Autodesk Inventor part; units mm, degrees
ref_plane "YZ Plane" through (0, 0, 0) normal (1, 0, 0) x (0, 1, 0)
ref_plane "XZ Plane" through (0, 0, 0) normal (0, 1, 0) x (-1, 0, 0)
ref_plane "XY Plane" through (0, 0, 0) normal (0, 0, 1) x (1, 0, 0)
sketch "Sketch2" plane through (0, 0, 0) normal (0, 1, 0) x (-1, 0, 0)
  line L0 (-49, 47) -> (-20, 47) construction
  line L1 (49, 47) -> (49, -47) construction
  line L2 (49, -47) -> (-49, -47)
  line L3 (-49, -47) -> (-49, 47) construction
  line L4 (-49, 47) -> (49, -47) construction
  line L5 (49, 47) -> (-49, -47) construction
  line L6 (49, -23) -> (45, -23)
  line L7 (45, -23) -> (45, 27)
  line L8 (45, 27) -> (49, 27)
  line L9 (49, 27) -> (49, -23)
  line L10 (-49, -23) -> (-45, -23)
  line L11 (-45, -23) -> (-45, 27)
  line L12 (-45, 27) -> (-49, 27)
  line L13 (-49, 27) -> (-49, -23)
  line L14 (25, -47) -> (-25, -47)
  line L15 (-25, -47) -> (-25, -43)
  line L16 (-25, -43) -> (25, -43)
  line L17 (25, -43) -> (25, -47)
  line L18 (0, -47) -> (0, 47)
  line L19 (49, 0) -> (-49, 0)
  line L20 (49, 2) -> (-45, 2) construction
  line L21 (20, 47) -> (0, 47) construction
  line L22 (-20, 47) -> (-20, 51) construction
  line L23 (-20, 51) -> (20, 51) construction
  line L24 (20, 51) -> (20, 47) construction
  line L25 (-20, 47) -> (20, 47)
  line L26 (0, 47) -> (-20, 47) construction
  line L27 (20, 47) -> (49, 47) construction
  line L28 (49, 43) -> (20, 43)
  line L29 (20, 43) -> (20, 47)
  line L30 (-49, 43) -> (-20, 43)
  line L31 (-20, 43) -> (-20, 47)
  line L32 (49, 43) -> (49, 27)
  line L33 (-49, 43) -> (-49, 27)
  line L34 (-49, -23) -> (-49, -47)
  line L35 (49, -23) -> (49, -47)
  point P0 (0, 0)
  point P1 (49, 27)
  point P2 (-49, 27)
  point P3 (0, 0)
  point P4 (0, 0)
  dimension "d7" = 98
  dimension "d8" = 94
  dimension "d5" = 4
  dimension "d6" = 50
  dimension "d3" = 4
  dimension "d4" = 50
  dimension "d1" = 50
  dimension "d2" = 4
  dimension "d0" = 2
  dimension "d27" = 4
  dimension "d28" = 40
  dimension "d31" = 4
extrude "Extrusion1" add sketch "Sketch2" along normal blind 4 contours L2 L17 L16 L18 L19 L7 L6 L35 | L2 L34 L10 L11 L19 L18 L16 L15 | L19 L18 L25 L29 L28 L32 L8 L7 | L19 L11 L12 L33 L30 L31 L25 L18
sketch "Sketch3" plane through (0, 4, 0) normal (0, 1, 0) x (1, 0, 0)
  circle A0 centre (0, 62.5) radius 11
  spline S0 degree 2 poles (-49, 47) (0, 109) (49, 47) knots 0 0 0 1 1 1
  circle A1 centre (66, -2) radius 7.5
  spline S1 degree 2 poles (49, 47) (117.0544, -3.4606) (49, -43) knots 0 0 0 1 1 1
  line L0 (0, 43) -> (0, -53.479) construction
  circle A2 centre (-66, -2) radius 7.5
  spline S2 degree 2 poles (-49, 47) (-117.0544, -3.4606) (-49, -43) knots 0 0 0 1 1 1
  line L1 (-66, 27) -> (-63.1716, 24.1716)
  line L2 (-63.1716, 24.1716) -> (-67.4142, 19.9289)
  line L3 (-67.4142, 19.9289) -> (-70.2426, 22.7574)
  line L4 (-70.2426, 22.7574) -> (-66, 27)
  line L5 (-20, -47) -> (-20, -51)
  line L6 (-20, -51) -> (20, -51)
  line L7 (20, -51) -> (20, -47)
  line L8 (49, 47) -> (25, 47) construction
  line L9 (25, 47) -> (25, 43)
  line L10 (25, 43) -> (-25, 43)
  line L11 (-25, 43) -> (-25, 47)
  line L12 (-25, 47) -> (-49, 47) construction
  line L13 (-49, 47) -> (-49, 23) construction
  line L14 (-49, 23) -> (-45, 23)
  line L15 (-45, 23) -> (-45, -27)
  line L16 (-45, -27) -> (-49, -27)
  line L17 (-49, -27) -> (-49, -43) construction
  line L18 (-49, -43) -> (-20, -43)
  line L19 (-20, -43) -> (-20, -47)
  line L20 (-20, -47) -> (20, -47)
  line L21 (20, -47) -> (20, -43)
  line L22 (20, -43) -> (49, -43)
  line L23 (49, -43) -> (49, -27) construction
  line L24 (49, -27) -> (45, -27)
  line L25 (45, -27) -> (45, 23)
  line L26 (45, 23) -> (49, 23)
  line L27 (49, 23) -> (49, 47) construction
  line L28 (-25, 43) -> (-25, 47)
  line L29 (-25, 47) -> (25, 47)
  line L30 (49, 23) -> (49, -27)
  line L31 (-49, 47) -> (-49, 23) construction
  line L32 (-49, -27) -> (-49, 23)
  line L33 (-45, 23) -> (-45, -27) construction
  line L34 (-45, -2) -> (45, -2) construction
  point P0 (0, 0)
  point P1 (0, 78)
  point P2 (83, -2)
  point P3 (-83, -2)
  point P4 (-49, -2)
  dimension "d12" = 22
  dimension "d14" = 15.5
  dimension "d18" = 15
  dimension "d19" = 17
  dimension "d21" = 6
  dimension "d22" = 4
  dimension "d29" = 20
  dimension "d33" = 15.5
  dimension "d34" = 17
  dimension "d35" = 4
  dimension "d36" = 45
  dimension "d37" = 17
extrude "Extrusion2" add sketch "Sketch3" against normal blind 4 contours S0 S1 L22 L21 L20 L19 L18 S2
sketch "Sketch4" plane through (0, 4, 0) normal (0, 1, 0) x (1, 0, 0)
  line L0 (16, 9) -> (20, 9)
  line L1 (20, 9) -> (20, 3)
  line L2 (20, 3) -> (16, 3)
  line L3 (16, 3) -> (16, 9)
  line L4 (16, -3) -> (20, -3)
  line L5 (20, -3) -> (20, -9)
  line L6 (20, -9) -> (16, -9)
  line L7 (16, -9) -> (16, -3)
  line L8 (-163.8761, 0) -> (163.8761, 0)
  line L9 (45, -27) -> (45, 23)
  point P0 (0, 0)
  dimension "d42" = 6
  dimension "d43" = 4
  dimension "d44" = 6
  dimension "d45" = 25
extrude "Extrusion3" cut sketch "Sketch4" against normal through all
properties part number "CarBottom_V3" material "Wood (Oak)"
Source: CAD feature listing. Evaluate the final solid. Frame: model axes, mm. A direction names the side the tool comes from. Give positions to 0.01 mm unless a question says otherwise; leave off trailing zeros. Return JSON: item names as keys, results as strings. Group by question number.
1) First-contact query: pin 1 Ø1 at (y, z) = (3, -28.5) entering from +X; pin 2 Ø1.2 at (y, z) = (1.5, 5.5) entering from +X; pin 3 Ø2 at (x, y) = (-33.5, 3) entering from +Z. Flat tips, straight axial feed; report the tip coordinate or a pass-through.
2) Ray query, L1, parallel to X at y = 1.8, z = 6.5; L2, parallel to X at y = 0.4, z = 25; L3, parallel to Z at x = -66, y = 1.9. Return the intervals inside material, ascending.
3) Cut plane A-A, the plane x = 0. Give the number of separate pieces and of enclosed holes in the cut face, then the cut area to 3 significant figures.
4) Draft query along Z for faces 1 (the face through (-65.263, 2.028, -22.08)), 2 (the face through (35, 2, 43)), 3 (the face through (-2, 0, -15)), 4 (the face through (18, 2, -9)). Return one class per face: released by +Z, released by -Z, zero draft, split by the parting line, or undercut.
5) Set-up query: faces 5 (the face through (20, 2, -6)), 6 (the face through (20, 2, 45)), 7 (the face through (0, 2, 47)). Return all of +Z, -Z, +X, -X, +Y, -Y with unobstructed straight access to the full face (end or side cutting, diameter ignored); none if empty.
Data:
{
 "1": {"pin 1": "stops at x = 70.14", "pin 2": "stops at x = 82.73", "pin 3": "stops at z = 43"},
 "2": {"L1": "x = -82.46 to -72, -60 to -49, -45 to 16, 20 to 45, 49 to 60, 72 to 82.46", "L2": "x = -72.42 to -49, -45 to 45, 49 to 72.42", "L3": "z = -32.47 to -27, -21.34 to -5.5, 9.5 to 31.2"},
 "3": {"separate pieces": "3", "enclosed holes": "0", "area": "396 mm²"},
 "4": {"face 1": "undercut", "face 2": "released by +Z", "face 3": "zero draft", "face 4": "undercut"},
 "5": {"face 5": "+Y, -Y", "face 6": "+Z, +X, +Y, -Y", "face 7": "+Z, +X, -X, +Y, -Y"}
}
